Check sheet for the modelled part. Datum: model origin and axes. Units: mm. Face numbers are marked on the shaded views. Round coordinates to 2 decimals unless told otherwise and drop trailing zeros. Order: outer loops, then holes, each group sorted by start corner. A loop starts at its lowest first (then second) coordinate and runs counter-clockwise, first axis right, second up. Notation, with made-up numbers: M 76,72.25 L 131,72.25 A6 cw 131,78.25 Z; hole C 64,-20.5 d2. An arc over 180 degrees is marked long. One line per item, written item: value. Start each with the question number.
(1) Cross-section at B-B, the plane x = 3.5. Enter the section's corners in (y, z), and give its area (3 significant figures).
(2) Depth check by flat-ended pin: pin 1 Ø10 at (x, z) = (2.5, 4.5) entering from -Y. Enter the tip coordinate at first touch or a pass-through.
(3) Release check for a two-part mould opening along Z. For the marked faces 1, 2 and 3 record: released by +Z, released by -Z, zero draft, split by the parting line, or undercut.
(4) Cross-section at C-C, the plane y = 3.2. Enter the section's corners in (x, z).
(5) Thickness scan on L1, parallel to Z at x = 55, y = 2.95; L2, parallel to X at y = 1, z = -0.75; L3, parallel to X at y = 2.7, z = -1. Record the ranges inside material, lowest first.
(6) Cross-section at A-A, the plane z = 0. Enter the section's corners in (x, y).
(7) Cross-section at D-D, the plane z = 4. Enter the section's corners in (x, y), and give its area (3 significant figures).
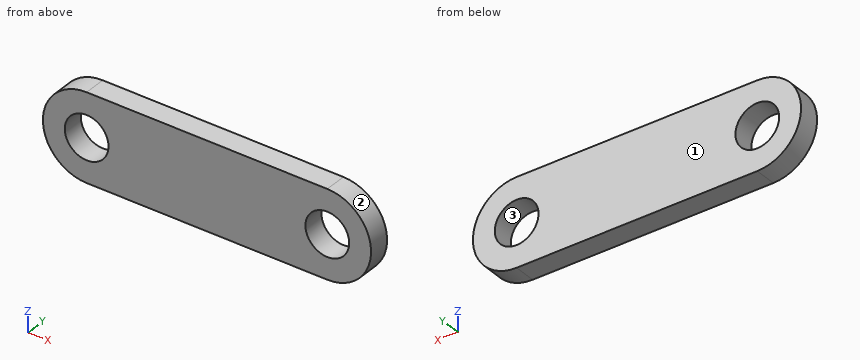
Autodesk Inventor part; units mm, degrees
ref_plane "YZ Plane" through (0, 0, 0) normal (1, 0, 0) x (0, 1, 0)
ref_plane "XZ Plane" through (0, 0, 0) normal (0, 1, 0) x (-1, 0, 0)
ref_plane "XY Plane" through (0, 0, 0) normal (0, 0, 1) x (1, 0, 0)
sketch "草圖3" plane through (0, 0, 0) normal (0, 1, 0) x (-1, 0, 0)
  line L0 (-65, 0) -> (10, 0) construction
  line L1 (-55, 10) -> (0, 10)
  line L2 (0, -10) -> (-55, -10)
  arc A0 (-55, 10) -> (-55, -10) centre (-55, 0) ccw
  arc A1 (0, -10) -> (0, 10) centre (0, 0) ccw
  circle A2 centre (-55, 0) radius 5
  circle A3 centre (0, 0) radius 5
  point P0 (-27.5, 0)
  dimension "hole" = 10
  dimension "d14" = 20
  dimension "center_distance" = 55
extrude "擠出3" add sketch "草圖3" along normal blind 5
equation "\"d14\" = 2 * hole"
properties part number "Binary link"
Values found:
1. outline: M 0,-10 L 5,-10 L 5,-3.57 L 0,-3.57 Z; M 0,3.57 L 5,3.57 L 5,10 L 0,10 Z
1. area: 64.3 mm^2
2. pin 1: y = 0
3. face 1: zero draft
3. face 2: split by the parting line
3. face 3: undercut
4. outline: M 0,-10 L 55,-10 A10 ccw 55,10 L 0,10 A10 ccw Z; hole C 0,0 d10; hole C 55,0 d10
5. L1: -10 to -5, 5 to 10
5. L2: -9.97 to -4.94, 4.94 to 50.06, 59.94 to 64.97
5. L3: -9.95 to -4.9, 4.9 to 50.1, 59.9 to 64.95
6. outline: M -10,0 L -5,0 L -5,5 L -10,5 Z; M 5,0 L 50,0 L 50,5 L 5,5 Z; M 60,0 L 65,0 L 65,5 L 60,5 Z
7. outline: M -9.17,0 L -3,0 L -3,5 L -9.17,5 Z; M 3,0 L 52,0 L 52,5 L 3,5 Z; M 58,0 L 64.17,0 L 64.17,5 L 58,5 Z
7. area: 307 mm^2
